from build123d import *

# Parameters (mm, degrees)
CROQUIS2_R              = 12.5
CROQUIS2_R_2            = 11
SALIENTE_EXTRUIR1_DEPTH = 10
SALIENTE_EXTRUIR2_DEPTH = 5
CROQUIS2_6_W            = 40
CROQUIS2_6_H            = 3
SALIENTE_EXTRUIR3_DEPTH = 40
CROQUIS2_7_W            = 40
CROQUIS2_7_H            = 3
SALIENTE_EXTRUIR4_DEPTH = 20


with BuildPart() as part:
    # Croquis2 → Saliente-Extruir1 (new body)
    with BuildSketch(Plane.XY):
        Circle(CROQUIS2_R)
        Circle(CROQUIS2_R_2, mode=Mode.SUBTRACT)
    extrude(amount=SALIENTE_EXTRUIR1_DEPTH)

    # Croquis2<4> → Saliente-Extruir2 (add)
    with BuildSketch(Plane.XY):
        with BuildLine():
            Line((-11.363241786, -5.208333333), (0, -30))
            Line((0, -30), (0, -27))
            Line((0, -27), (40, -27))
            ThreePointArc((40, -27), (21.826404492, -18.005513943), (12.5, 0))
            ThreePointArc((12.5, 0), (2.665471597, -12.212504295), (-11.363241786, -5.208333333))
        make_face()
    extrude(amount=SALIENTE_EXTRUIR2_DEPTH)

    # Croquis2<6> → Saliente-Extruir3 (add)
    with BuildSketch(Plane.XY):
        with Locations((20, -28.5)):
            Rectangle(CROQUIS2_6_W, CROQUIS2_6_H)
    extrude(amount=SALIENTE_EXTRUIR3_DEPTH)


with BuildPart() as body_2:
    # Simetría2: mirrored copy
    add(part.part.mirror(Plane(origin=(0, 0, -10), x_dir=(1, 0, 0), z_dir=(0, 0, -1))))


with BuildPart() as part_1:
    add(part.part)

    add(body_2.part)  # Saliente-Extruir4 merges body 2
    # Croquis2<7> → Saliente-Extruir4 (add)
    with BuildSketch(Plane.XY):
        with Locations((20, -28.5)):
            Rectangle(CROQUIS2_7_W, CROQUIS2_7_H)
    extrude(amount=-SALIENTE_EXTRUIR4_DEPTH)


solid = part_1.part
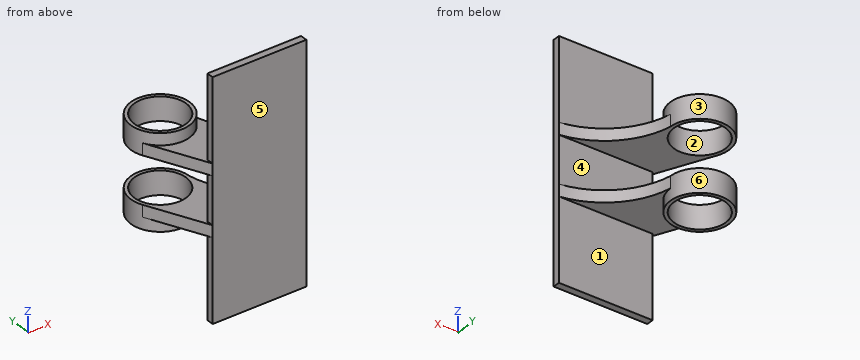
The model under review builds one solid part; all positions refer to its coordinate system, in mm. Face numbers are marked on the shaded views. A direction names the side the tool comes from. Round coordinates to 2 decimals unless told otherwise and drop trailing zeros. Loops run counter-clockwise (first coordinate to the right, second up) from the corner with the lowest first, then second, coordinate; pieces in that order, holes last. Notation, with made-up numbers: (-25, -20) -> (-18, -20) arc R32 ccw to (-18, 8) -> close; hole circle Ø3 at (64, 26.5). An arc over 180 degrees is marked (long way). Write item = value, one per line. Start each with the question number.
Item 1: Take a section at D-D on y = -18.5. Give the boundary of the cut face in (x, z), plus the area to 3 significant figures.
Item 2: Mouldability with a two-part tool opening along X and no side actions: class the marked faces 1, 2 and 3 as released by +X, released by -X, zero draft, split by the parting line, or undercut.
Item 3: Take a section at B-B on x = 24. Give the boundary of the cut face in (y, z).
Item 4: Take a section at A-A on y = 2. Give the boundary of the cut face in (x, z).
Item 5: To check wall thickness, follow L1, parallel to Y at x = 0, z = -22; L2, parallel to Z at x = 22.5, y = -19; L3, parallel to Z at x = 11, y = 3. State the ranges of each line that lie inside material, in increasing order.
Item 6: For the marked faces 4, 5 and 6, list the 3-axis set-ups (+Z, -Z, +X, -X, +Y, -Y) from which the entire face can be reached by the end or side of a thin tool; tool diameter is ignored.
Item 7: Take a section at C-C on z = 23.5. Give the boundary of the cut face in (x, y).
Item 8: Insertion check: pin 1 (10 mm diameter, centred on y = -17.5, z = 6, fed in from +X); pin 2 (1.5 mm diameter, centred on y = -29, z = -45.5, fed in from -X); pin 3 (10.5 mm diameter, centred on x = 23, z = -36, fed in from +Y); pin 4 (12.5 mm diameter, centred on x = -3.5, y = 2, fed in from +Z). Each pin has a flat end and moves straight along its axis. Give the tip position at first contact, or say it passes through.
Result:
q1.outline = (-5.27, -25) -> (22.34, -25) -> (22.34, -20) -> (-5.27, -20) -> close; (-5.27, 0) -> (22.34, 0) -> (22.34, 5) -> (-5.27, 5) -> close
q1.area = 276 mm²
q2.face_1 = zero draft
q2.face_2 = undercut
q2.face_3 = split by the parting line
q3.outline = (-30, -60) -> (-27, -60) -> (-27, -25) -> (-19.96, -25) -> (-19.96, -20) -> (-27, -20) -> (-27, 0) -> (-19.96, 0) -> (-19.96, 5) -> (-27, 5) -> (-27, 40) -> (-30, 40) -> close
q4.outline = (-12.34, -30) -> (-10.82, -30) -> (-10.82, -20) -> (-12.34, -20) -> close; (-12.34, 0) -> (-10.82, 0) -> (-10.82, 10) -> (-12.34, 10) -> close; (10.82, -30) -> (12.34, -30) -> (12.34, -20) -> (10.82, -20) -> close; (10.82, 0) -> (12.34, 0) -> (12.34, 10) -> (10.82, 10) -> close
q5.L1 = -30 to -11, 11 to 12.5
q5.L2 = -25 to -20, 0 to 5
q5.L3 = -30 to -20, 0 to 10
q6.face_4 = +X, -X, +Y
q6.face_5 = +Z, -Z, +X, -X, -Y
q6.face_6 = -Z
q7.outline = (0, -30) -> (40, -30) -> (40, -27) -> (0, -27) -> close
q8.pin_1 = 27.41
q8.pin_2 = 0
q8.pin_3 = -27
q8.pin_4 = through
